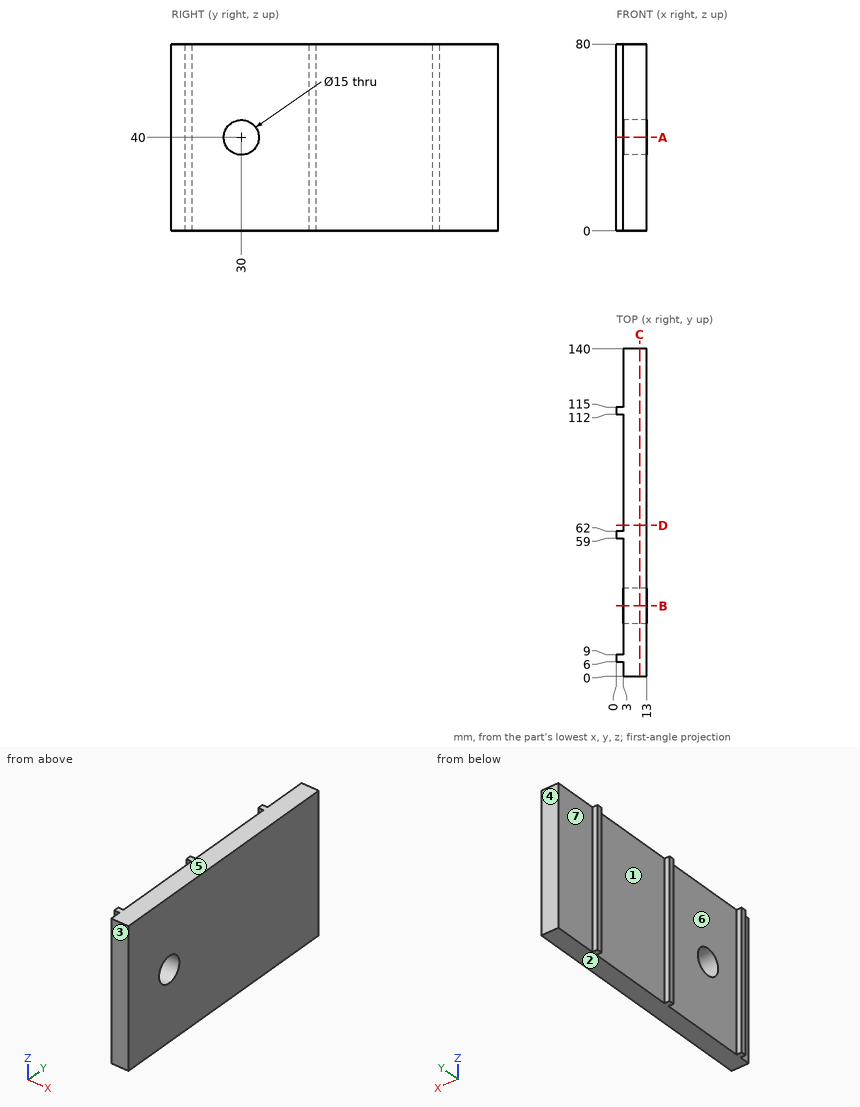
For this review, use the dimensioned drawing (mm, ordinates from the lowest corner) and the shaded views. A direction names the side the tool comes from. Round coordinates to 2 decimals unless told otherwise and drop trailing zeros. Write each loop counter-clockwise with the first axis right and the second up, starting at its lowest first coordinate (ties: lowest second). Pieces come first, ordered by that corner, then holes. Notation, with made-up numbers: M -16,48.5 L -4,48.5 A9 cw -4,58.5 Z; hole C 81.5,35.5 d6. An arc over 180 degrees is marked long. Use CSV: the item, a comma, the result in double quotes. Start each with the question number.
(1) We need section B-B, the plane y = 30. State the section outline as (x, z) points, then the cut area to 3 significant figures.
(2) For line 1 along Y through (x, z) = (2.75, 62.5); line 2 along Z through (x, y) = (7.75, 30); line 3 along Z through (x, y) = (11.75, 25), list the stretches that pass through material, from the lowest coordinate up.
(3) Tool access review of the marked faces 5, 6 and 7: name each direction out of +Z, -Z, +X, -X, +Y, -Y from which nothing blocks a thin tool from reaching the whole face with its end or side.
(4) We need section D-D, the plane y = 64.5. State the section outline as (x, z) points, then the cut area to 3 significant figures.
(5) Clearance check with flat-ended pins moving along their axes: P1, Ø12.5, axis at y = 121.5, z = 21.5, coming from the -X side; P2, Ø0.9, axis at x = 1, z = 38, coming from the -Y side; P3, Ø2.5, axis at x = 1, z = 31, coming from the +Y side. State where each tip first meets the part, or that it passes through.
(6) We need section C-C, the plane x = 10. State the section outline as (y, z) points.
(7) The part is to be moulded in two halves that separate along Y. For the marked faces 1, 2, 3 and 4, say which applies: +Y half, -Y half, draft (parallel to the pull), parting line (faces both ways), or undercut.
(8) We need section A-A, the plane z = 40. State the section outline as (x, y) points.
Findings:
1,outline,"M 3,0 L 13,0 L 13,32.5 L 3,32.5 Z; M 3,47.5 L 13,47.5 L 13,80 L 3,80 Z"
1,area,"650 mm^2"
2,line 1,"6 to 9, 59 to 62, 112 to 115"
2,line 2,"0 to 32.5, 47.5 to 80"
2,line 3,"0 to 34.41, 45.59 to 80"
3,face 5,"+Z, +X, -X, +Y, -Y"
3,face 6,"+Z, -Z, -X"
3,face 7,"+Z, -Z, -X, +Y"
4,outline,"M 3,0 L 13,0 L 13,80 L 3,80 Z"
4,area,"800 mm^2"
5,P1,"x = 3"
5,P2,"y = 6"
5,P3,"y = 115"
6,outline,"M 0,0 L 140,0 L 140,80 L 0,80 Z; hole C 30,40 d15"
7,face 1,"undercut"
7,face 2,"draft"
7,face 3,"-Y half"
7,face 4,"+Y half"
8,outline,"M 0,6 L 3,6 L 3,0 L 13,0 L 13,22.5 L 3,22.5 L 3,9 L 0,9 Z; M 0,59 L 3,59 L 3,37.5 L 13,37.5 L 13,140 L 3,140 L 3,115 L 0,115 L 0,112 L 3,112 L 3,62 L 0,62 Z"
